Geometry check sheet. Reference: the model listing, model coordinates, mm. Face numbers are marked on the shaded views. Round coordinates to 2 decimals unless told otherwise and drop trailing zeros. Loops run counter-clockwise (first coordinate to the right, second up) from the corner with the lowest first, then second, coordinate; pieces in that order, holes last. Notation, with made-up numbers: M 65.5,-35 L 102.5,-35 A10 ccw 102.5,-30 Z; hole C 47.25,42 d6. An arc over 180 degrees is marked long. Use one line per item in the form item = value. Start each with the question number.
1. Draft check along Y on the marked faces 1, 2 and 3. Enter one of: pulls with the +Y half, pulls with the -Y half, needs draft (parallel to the pull), parting line crosses it, or undercut.
2. Cross-section at C-C (x = 1.25). Record the boundary of the cut face in (y, z).
3. Cross-section at A-A (y = 0). Record the boundary of the cut face in (x, z), then the cut area to 3 significant figures.
4. Cross-section at B-B (z = 6.75). Record the boundary of the cut face in (x, y).
5. Cross-section at D-D (z = 16). Record the boundary of the cut face in (x, y), then the cut area to 3 significant figures.
6. Material ranges on line 1 (Y direction, x = 0, z = 5.25); line 2 (Z direction, x = -5.5, y = 3), recorded low to high.
```python
from build123d import *

# Parameters (mm, degrees)
SKETCH1_W           = 20
SKETCH1_H           = 20
BOSS_EXTRUDE1_DEPTH = 20
SKETCH2_R           = 5
CUT_EXTRUDE1_DEPTH  = 20
SKETCH3_R           = 5
CUT_EXTRUDE2_DEPTH  = 20


with BuildPart() as part:
    # Sketch1 → Boss-Extrude1 (new body)
    with BuildSketch(Plane.XY):
        Rectangle(SKETCH1_W, SKETCH1_H)
    extrude(amount=BOSS_EXTRUDE1_DEPTH)

    # Sketch2 → Cut-Extrude1 (cut)
    with BuildSketch(Plane.XY.offset(20)):
        Circle(SKETCH2_R)
    extrude(amount=-CUT_EXTRUDE1_DEPTH, mode=Mode.SUBTRACT)

    # Sketch3 → Cut-Extrude2 (cut)
    with BuildSketch(Plane(origin=(10, 0, 0), x_dir=(0, 0, -1), z_dir=(1, 0, 0))):
        with Locations((-10, 0)):
            Circle(SKETCH3_R)
    extrude(amount=-CUT_EXTRUDE2_DEPTH, mode=Mode.SUBTRACT)


solid = part.part
```
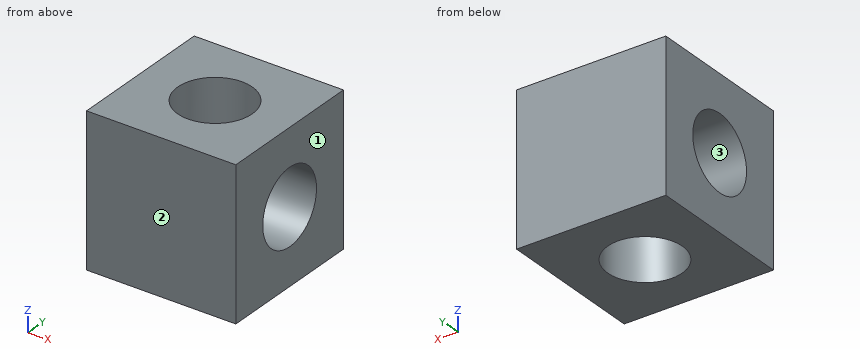
Reported:
q1.face_1 = needs draft
q1.face_2 = pulls with the -Y half
q1.face_3 = undercut
q2.outline = M -10,0 L -4.84,0 L -4.84,8.75 A5 cw -4.84,11.25 L -4.84,20 L -10,20 Z; M 4.84,0 L 10,0 L 10,20 L 4.84,20 L 4.84,11.25 A5 cw 4.84,8.75 Z
q3.outline = M -10,0 L -5,0 L -5,5 L -10,5 Z; M -10,15 L -5,15 L -5,20 L -10,20 Z; M 5,0 L 10,0 L 10,5 L 5,5 Z; M 5,15 L 10,15 L 10,20 L 5,20 Z
q3.area = 100 mm²
q4.outline = M -10,-10 L 10,-10 L 10,-3.8 L 3.25,-3.8 A5 cw -3.25,-3.8 L -10,-3.8 Z; M -10,3.8 L -3.25,3.8 A5 cw 3.25,3.8 L 10,3.8 L 10,10 L -10,10 Z
q5.outline = M -10,-10 L 10,-10 L 10,10 L -10,10 Z; hole C 0,0 d10
q5.area = 321 mm²
q6.line_1 = -10 to -5, 5 to 10
q6.line_2 = 0 to 6, 14 to 20
